Answer from the drawing. Dimensions are ordinates in mm from the lowest x, y and z of the part. A direction names the side the tool comes from. Round coordinates to 2 decimals unless told otherwise and drop trailing zeros. Loops run counter-clockwise (first coordinate to the right, second up) from the corner with the lowest first, then second, coordinate; pieces in that order, holes last. Notation, with made-up numbers: M 68,6 L 110,6 A24 cw 110,45 Z; hole C 16.25,4 d7. An arc over 180 degrees is marked long. Answer as CSV lines item,"result".
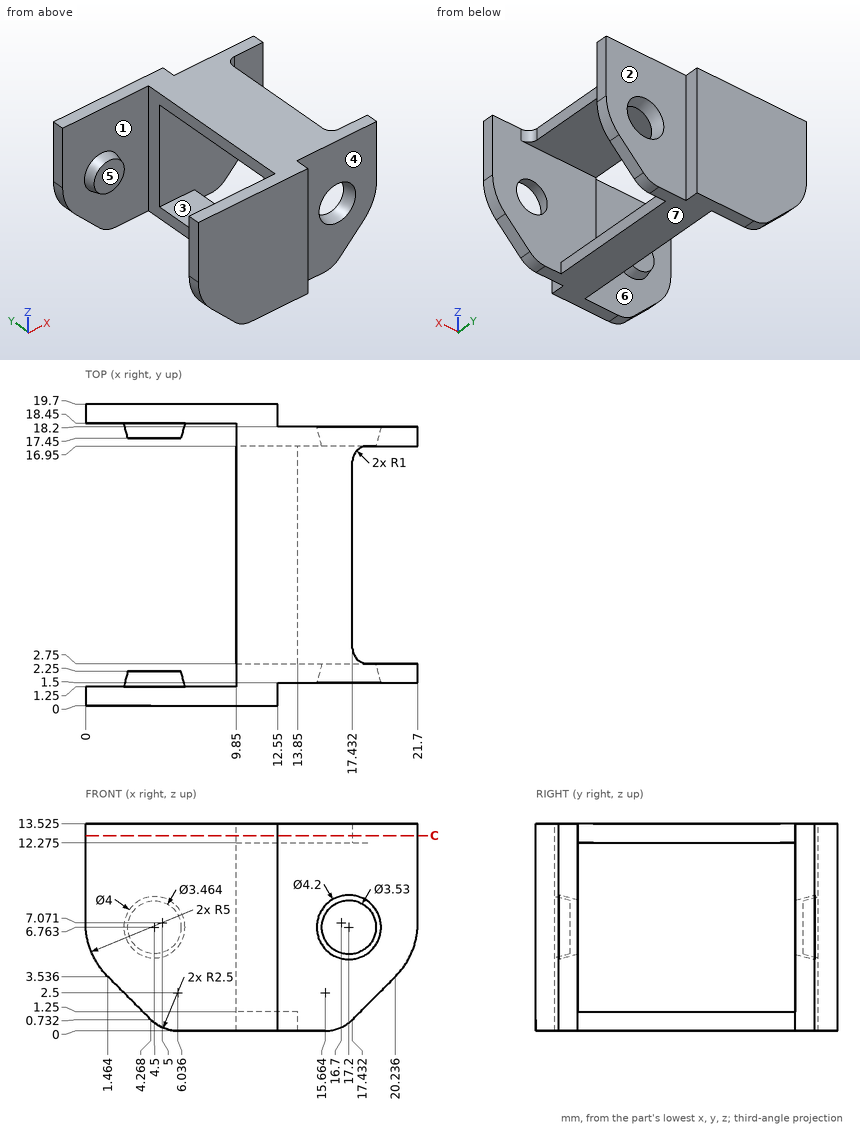
1) Each of these flat-tipped pins is pushed along its axis until it touches: P1, Ø2.5, axis at x = 16, y = 11, coming from the -Z side (1 decimal); P2, Ø0.6, axis at y = 11.5, z = 0.5, coming from the +X side; P3, Ø3, axis at y = 14, z = 10.5, coming from the -X side (3 decimals); P4, Ø1, axis at y = 10.5, z = 13, coming from the +X side. Where does it stop, or does it pass through?
Evaluation:
P1,"stops at z = 12.3"
P2,"stops at x = 13.85"
P3,"passes through"
P4,"stops at x = 17.43"
2) Determine the mould class of the marked faces 6 and 7 for opening direction X: released by +X, released by -X, zero draft, split by the parting line, or undercut.
Evaluation:
face 6,"undercut"
face 7,"zero draft"
3) Find section C-C, the plane z = 12.75. Give the vertices of the cut face in (x, y).
Evaluation:
outline,"M 0,0 L 12.55,0 L 12.55,1.5 L 21.7,1.5 L 21.7,2.75 L 18.43,2.75 A1 cw 17.43,3.75 L 17.43,15.95 A1 cw 18.43,16.95 L 21.7,16.95 L 21.7,18.2 L 12.55,18.2 L 12.55,19.7 L 0,19.7 L 0,18.45 L 9.85,18.45 L 9.85,1.25 L 0,1.25 Z"
4) Straight lines are drawn through the part: line 1 (Y direction, x = 11.25, z = 2); line 2 (Y direction, x = 6.25, z = 4.5); line 3 (Z direction, x = 16.75, y = 13.75) (1 decimal). For each, find the intervals that lie inside material, in ascending order.
Evaluation:
line 1,"y = 0 to 2.75, 16.95 to 19.7"
line 2,"y = 0 to 1.25, 18.45 to 19.7"
line 3,"z = 12.3 to 13.5"
5) A tool of negligible diameter and unlimited length cuts with its end or side. For the marked faces 1, 2, 3, 4 and 5, from which of +Z, -Z, +X, -X, +Y, -Y can it reach the whole face along a straight path? Write none if from no direction.
Evaluation:
face 1,"none"
face 2,"+Z, -Z, +X, +Y"
face 3,"+X, -X"
face 4,"+Z, -Z, +X, -Y"
face 5,"+Z, -Z, -X"
